from build123d import *

# Parameters (mm, degrees)
F1_W          = 152.0064324141
F1_H          = 151.6206115484
F3_DEPTH      = 50
F3_DEPTH_BACK = 50
F0_W          = 152.1505489945
F0_H          = 151.9152671099
F4_DEPTH      = 50
F4_DEPTH_BACK = 50
F2_W          = 152.4115279317
F2_H          = 151.8903151155
F5_DEPTH      = 50
F5_DEPTH_BACK = 50


# Not quite as in the source:
# - the program builds the solid bodies; features that only make, move or delete a surface that nothing else refers to are left out


with BuildPart() as f3:
    # F1 (on Top) → F3 (new body, two sides)
    with BuildSketch(Plane.XY) as f3_sk:
        with Locations((-0.0777542591, -0.7124021649)):
            Rectangle(F1_W, F1_H)
    extrude(amount=F3_DEPTH)
    extrude(f3_sk.sketch, amount=-F3_DEPTH_BACK)

    # F0 (on Front) → F4 (join, two sides)
    with BuildSketch(Plane.XZ) as f4_sk:
        with Locations((0.5021430552, -0.6082579494)):
            Rectangle(F0_W, F0_H)
    extrude(amount=F4_DEPTH)
    extrude(f4_sk.sketch, amount=-F4_DEPTH_BACK)

    # F2 (on Right) → F5 (join, two sides)
    with BuildSketch(Plane.YZ) as f5_sk:
        with Locations((-0.9317584336, 0.2604238689)):
            Rectangle(F2_W, F2_H)
    extrude(amount=F5_DEPTH)
    extrude(f5_sk.sketch, amount=-F5_DEPTH_BACK)


solid = f3.part
CAD build for the part. Positions are in the model's coordinates, mm. A direction names the side the tool comes from. Give positions to 0.01 mm unless a question says otherwise; leave off trailing zeros. Write each loop counter-clockwise with the first axis right and the second up, starting at its lowest first coordinate (ties: lowest second). Pieces come first, ordered by that corner, then holes. Notation, with made-up numbers: (30.25, -5.75) - (48.25, -5.75) arc R24 cw to (48.25, 24.25) - close; hole circle Ø11 at (-19.75, 7). An arc over 180 degrees is marked (long way). Answer as CSV lines item,"result".
Q1. Flat gauge pins, fed straight in: pin 1 Ø12.5 at (x, y) = (65.5, 60.5) entering from -Z; pin 2 Ø13 at (x, z) = (-60.5, -22.5) entering from +Y; pin 3 Ø20.5 at (x, y) = (62.5, -64.5) entering from +Z. Where does each tip first touch, or does it go through?
Result set:
pin 1,"z = -50"
pin 2,"y = 75.1"
pin 3,"z = 50"
Q2. Band-saw the part on B-B (y = -63.5). Give the cut face in (x, z).
Result set:
outline,"(-76.08, -50) - (-50, -50) - (-50, -75.68) - (50, -75.68) - (50, -50) - (75.93, -50) - (75.93, 50) - (50, 50) - (50, 76.21) - (-50, 76.21) - (-50, 50) - (-76.08, 50) - close"
Q3. Drill centre lines: line 1 (X direction, y = 28, z = -61.5); line 2 (X direction, y = -57.5, z = -31); line 3 (Z direction, x = -56.5, y = -58). Where is each one in solid material? Low to high. Write a range as from..to.
Result set:
line 1,"-75.57..76.58"
line 2,"-76.08..75.93"
line 3,"-50..50"
Q4. 3-axis set-ups, long thin cutter, end or side, ignore diameter. For faces 1 (the face through (-63, 50, 63)), 2 (the face through (75.925, 62, 1)), 3 (the face through (-63, -1, 75.349)): which of +Z, -Z, +X, -X, +Y, -Y reach the whole face in a straight line?
Result set:
face 1,"+Z, -X, +Y"
face 2,"+Z, -Z, +X, +Y"
face 3,"+Z, -X, +Y, -Y"
Q5. Band-saw the part on A-A (x = 66). Give the cut face in (y, z).
Result set:
outline,"(-76.52, -50) - (-50, -50) - (-50, -76.57) - (50, -76.57) - (50, -50) - (75.1, -50) - (75.1, 50) - (50, 50) - (50, 75.35) - (-50, 75.35) - (-50, 50) - (-76.52, 50) - close"
